from build123d import *

# Parameters (mm, degrees)
SKETCH1_W           = 100
SKETCH1_H           = 85
BOSS_EXTRUDE1_DEPTH = 5
SKETCH4_W           = 100
SKETCH4_H           = 85
SKETCH4_W_2         = 96
SKETCH4_H_2         = 81
BOSS_EXTRUDE3_DEPTH = 10
FILLET1_R           = 5
FILLET2_R           = 3
SKETCH8_W           = 45.72
SKETCH8_H           = 30
CUT_EXTRUDE3_DEPTH  = 2.5
SKETCH9_W           = 41.72
SKETCH9_H           = 26
CUT_EXTRUDE4_DEPTH  = 100


with BuildPart() as part:
    # Sketch1 → Boss-Extrude1 (new body)
    with BuildSketch(Plane.XY):
        Rectangle(SKETCH1_W, SKETCH1_H)
    extrude(amount=BOSS_EXTRUDE1_DEPTH)

    # Sketch4 → Boss-Extrude3 (add)
    with BuildSketch(Plane(origin=(0, 0, 0), x_dir=(-1, 0, 0), z_dir=(0, 0, -1))):
        Rectangle(SKETCH4_W, SKETCH4_H)
        Rectangle(SKETCH4_W_2, SKETCH4_H_2, mode=Mode.SUBTRACT)
    extrude(amount=-BOSS_EXTRUDE3_DEPTH)

    # Fillet1
    fillet1_edges = [part.edges().sort_by_distance(p)[0] for p in [
        (50, -42.5, 5),
        (-50, -42.5, 5),
        (-50, 42.5, 5),
        (50, 42.5, 5),
    ]]
    fillet(fillet1_edges, radius=FILLET1_R)

    # Fillet2
    fillet2_edges = [part.edges().sort_by_distance(p)[0] for p in [
        (0, -42.5, 0),
        (50, 0, 0),
        (-50, 0, 0),
        (0, 42.5, 0),
        (-48.535533906, 41.035533906, 0),
        (48.535533906, 41.035533906, 0),
        (48.535533906, -41.035533906, 0),
        (-48.535533906, -41.035533906, 0),
    ]]
    fillet(fillet2_edges, radius=FILLET2_R)

    # Sketch8 → Cut-Extrude3 (cut)
    with BuildSketch(Plane(origin=(0, 0, 0), x_dir=(-1, 0, 0), z_dir=(0, 0, -1))):
        with Locations((-19.14, -19.5)):
            Rectangle(SKETCH8_W, SKETCH8_H)
    extrude(amount=-CUT_EXTRUDE3_DEPTH, mode=Mode.SUBTRACT)

    # Sketch9 → Cut-Extrude4 (cut)
    with BuildSketch(Plane(origin=(0, 0, 2.5), x_dir=(-1, 0, 0), z_dir=(0, 0, -1))):
        with Locations((-19.14, -19.5)):
            Rectangle(SKETCH9_W, SKETCH9_H)
    extrude(amount=-CUT_EXTRUDE4_DEPTH, mode=Mode.SUBTRACT)


solid = part.part
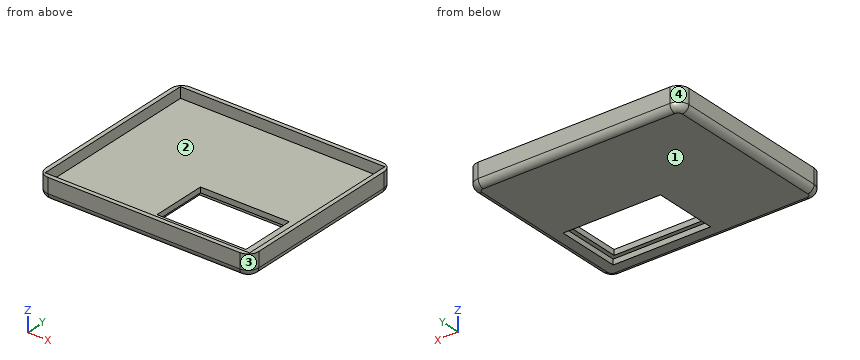
CAD build for the part. Positions are in the model's coordinates, mm. Face numbers are marked on the shaded views. Give positions to 0.01 mm unless a question says otherwise; leave off trailing zeros. Write each loop counter-clockwise with the first axis right and the second up, starting at its lowest first coordinate (ties: lowest second). Pieces come first, ordered by that corner, then holes. Notation, with made-up numbers: (-7.5, 82) -> (19.5, 82) arc R22 ccw to (19.5, 101) -> close; hole circle Ø1 at (-18, 71). An arc over 180 degrees is marked (long way). Return JSON: item names as keys, results as strings.
Item 1: Two-plate mould, pull along X, no slides. Class the marked faces 1, 2, 3 and 4: +X half, -X half, draft (parallel to the pull), parting line (faces both ways), or undercut.
Answer below:
{"face 1": "draft", "face 2": "undercut", "face 3": "+X half", "face 4": "-X half"}
Item 2: Drop flat-ended pins along their axis: pin 1 (2 mm diameter, centred on x = 24, z = 1.5, fed in from +Y); pin 2 (2 mm diameter, centred on y = -21.5, z = 1.5, fed in from -X); pin 3 (1.2 mm diameter, centred on y = -15, z = 1.5, fed in from +X). Give the stop position or say it passes through.
Answer below:
{"pin 1": "stops at y = 42.46", "pin 2": "stops at x = -49.96", "pin 3": "stops at x = 49.86"}
Item 3: Band-saw the part on C-C (x = 2.5). List the corners of the cut face in (y, z).
Answer below:
{"outline": "(-42.5, 3) arc R3 ccw to (-39.5, 0) -> (-34.5, 0) -> (-34.5, 2.5) -> (-32.5, 2.5) -> (-32.5, 5) -> (-40.5, 5) -> (-40.5, 10) -> (-42.5, 10) -> close; (-6.5, 2.5) -> (-4.5, 2.5) -> (-4.5, 0) -> (39.5, 0) arc R3 ccw to (42.5, 3) -> (42.5, 10) -> (40.5, 10) -> (40.5, 5) -> (-6.5, 5) -> close"}
Item 4: Band-saw the part on D-D (y = 14). List the corners of the cut face in (x, z), then the cut area to 3 significant figures.
Answer below:
{"outline": "(-50, 3) arc R3 ccw to (-47, 0) -> (47, 0) arc R3 ccw to (50, 3) -> (50, 10) -> (48, 10) -> (48, 5) -> (-48, 5) -> (-48, 10) -> (-50, 10) -> close", "area": "516 mm2"}
Item 5: Band-saw the part on B-B (z = 8.5). List the corners of the cut face in (x, y), then the cut area to 3 significant figures.
Answer below:
{"outline": "(-50, -37.5) arc R5 ccw to (-45, -42.5) -> (45, -42.5) arc R5 ccw to (50, -37.5) -> (50, 37.5) arc R5 ccw to (45, 42.5) -> (-45, 42.5) arc R5 ccw to (-50, 37.5) -> close; hole (-48, -40.5) -> (48, -40.5) -> (48, 40.5) -> (-48, 40.5) -> close", "area": "703 mm2"}
Item 6: Drill centre lines: probe 1 along Y at (x, z) = (2, 5.75); probe 2 along Y at (x, z) = (29, 4.5); probe 3 along X at (y, z) = (-16.5, 9.25). Where is each one in solid material? Low to high.
Answer below:
{"probe 1": "y = -42.5 to -40.5, 40.5 to 42.5", "probe 2": "y = -42.5 to -32.5, -6.5 to 42.5", "probe 3": "x = -50 to -48, 48 to 50"}
Item 7: Band-saw the part on A-A (y = -11.5). List the corners of the cut face in (x, z).
Answer below:
{"outline": "(-50, 3) arc R3 ccw to (-47, 0) -> (-3.72, 0) -> (-3.72, 2.5) -> (-1.72, 2.5) -> (-1.72, 5) -> (-48, 5) -> (-48, 10) -> (-50, 10) -> close; (40, 2.5) -> (42, 2.5) -> (42, 0) -> (47, 0) arc R3 ccw to (50, 3) -> (50, 10) -> (48, 10) -> (48, 5) -> (40, 5) -> close"}
